from build123d import *

# Parameters (mm, degrees)
POCKET_DEPTH       = 5.2
POCKET001_DEPTH    = 131.2836295795
POLARPATTERN_COUNT = 3
SKETCH003_R        = 1.65
POCKET002_DEPTH    = 3.601


with BuildPart() as part:
    # Sketch → Revolution (revolve)
    with BuildSketch(Plane.XZ):
        Polygon((15.1, 0), (15.1, 3.9), (21.6, 3.9), (21.6, 1.7), (22.6, 1.7), (22.6, 0), align=None)
    revolve(axis=Axis((0, 0, 0), (0, 0, 1)))

    # Sketch001 → Pocket (cut)
    with BuildSketch(Plane.XY.offset(0.3)):
        with BuildLine():
            ThreePointArc((-15.9712383567, -3.8204989231), (-18.8447644437, -5.9331508585), (-16.9057454793, -8.9265863145))
            ThreePointArc((-16.1835232571, -10.1775118978), (-16.2776050381, -9.3978796505), (-16.9057454793, -8.9265863145))
            ThreePointArc((-16.1835232571, -10.1775118978), (-14.5606415898, -13.3534693073), (-11.2942683009, -11.9212486852))
            ThreePointArc((-9.7295516419, -11.5475462696), (-10.6061902717, -11.3396396422), (-11.2942683009, -11.9212486852))
            ThreePointArc((-9.7295516419, -11.5475462696), (0, -15.1), (9.7295516419, -11.5475462696))
            ThreePointArc((11.2942683009, -11.9212486852), (10.6061902717, -11.3396396422), (9.7295516419, -11.5475462696))
            ThreePointArc((11.2942683009, -11.9212486852), (14.5606415898, -13.3534693073), (16.1835232571, -10.1775118978))
            ThreePointArc((16.9057454793, -8.9265863145), (16.2776050381, -9.3978796505), (16.1835232571, -10.1775118978))
            ThreePointArc((16.9057454793, -8.9265863145), (18.8447644437, -5.9331508585), (15.9712383567, -3.8204989231))
            ThreePointArc((14.8652442418, -2.6522657545), (15.1235111358, -3.5154103916), (15.9712383567, -3.8204989231))
            ThreePointArc((14.8652442418, -2.6522657545), (13.0769835971, 7.55), (5.1356925999, 14.1998120241))
            ThreePointArc((4.6769700558, 15.7417476083), (4.517320864, 14.8550500338), (5.1356925999, 14.1998120241))
            ThreePointArc((4.6769700558, 15.7417476083), (4.2841228539, 19.2866201659), (0.7222222222, 19.1040982123))
            ThreePointArc((-0.7222222222, 19.1040982123), (0, 18.7957593011), (0.7222222222, 19.1040982123))
            ThreePointArc((-0.7222222222, 19.1040982123), (-4.2841228539, 19.2866201659), (-4.6769700558, 15.7417476083))
            ThreePointArc((-5.1356925999, 14.1998120241), (-4.517320864, 14.8550500338), (-4.6769700558, 15.7417476083))
            ThreePointArc((-5.1356925999, 14.1998120241), (-13.0769835972, 7.55), (-14.8652442418, -2.6522657545))
            ThreePointArc((-15.9712383567, -3.8204989231), (-15.1235111358, -3.5154103916), (-14.8652442418, -2.6522657545))
        make_face()
    extrude(amount=POCKET_DEPTH, mode=Mode.SUBTRACT)

    # Sketch002 → Pocket001 (cut, through all)
    with BuildSketch(Plane.XY.offset(0.7)):
        with BuildLine():
            Line((-21.1456411257, 3.728513813), (-19.8005265105, 3.4913338142))
            ThreePointArc((-19.8005265105, 3.4913338142), (-17.143892895, 3.9448230849), (-15.3779467169, 5.9806985187))
            ThreePointArc((-8.5602136605, 14.1057698155), (-12.6397419459, 10.6059852697), (-15.3779467169, 5.9806985187))
            ThreePointArc((-8.5602136605, 14.1057698155), (-6.8619255723, 16.1984130552), (-6.876646489, 18.8934309501))
            Line((-7.3438021199, 20.1769304973), (-6.876646489, 18.8934309501))
            ThreePointArc((-6.6329850074, 21.6047103635), (-7.2948567632, 21.0433924702), (-7.3438021199, 20.1769304973))
            ThreePointArc((-6.6329850074, 21.6047103635), (-17.3126154887, 14.5269867812), (-22.428296266, 2.7805622822))
            ThreePointArc((-21.1456411257, 3.728513813), (-21.9904400194, 3.5298512156), (-22.428296266, 2.7805622822))
        make_face()
    pocket001 = extrude(amount=POCKET001_DEPTH, mode=Mode.SUBTRACT)

    # PolarPattern: Pocket001 ×3 about axis
    polarpattern_axis = Axis((0, 0, 0.7), (0, 0, 1))
    for i in range(1, POLARPATTERN_COUNT):
        add(pocket001.rotate(polarpattern_axis, i * 360 / POLARPATTERN_COUNT), mode=Mode.SUBTRACT)

    # Sketch003 → Pocket002 (cut, through all)
    with BuildSketch(Plane.XY.offset(0.3)):
        with Locations((8.75, 15.1554445662)):
            Circle(SKETCH003_R)
        with Locations((-17.5, 0)):
            Circle(SKETCH003_R)
        with Locations((8.75, -15.1554445662)):
            Circle(SKETCH003_R)
    extrude(amount=POCKET002_DEPTH, mode=Mode.SUBTRACT)


solid = part.part
Can you work these out from the model? Positions are in its coordinate system, mm. A direction names the side the tool comes from. Give positions to 0.01 mm unless a question says otherwise; leave off trailing zeros. Loops run counter-clockwise (first coordinate to the right, second up) from the corner with the lowest first, then second, coordinate; pieces in that order, holes last. Notation, with made-up numbers: (64, -20.75) - (111, -20.75) arc R26 cw to (111, 2.25) - close; hole circle Ø11 at (70, 64). An arc over 180 degrees is marked (long way). Return JSON: item names as keys, results as strings.
1. I'm going to push flat-ended pins straight in: pin 1 Ø3 at (x, y) = (-17.5, 0) entering from +Z; pin 2 Ø3 at (x, y) = (18, 10.5) entering from +Z; pin 3 Ø2 at (y, z) = (-11, 2) entering from -X. Where does each tip first touch, or does it pass through?
Output values:
{"pin 1": "stops at z = 0.3", "pin 2": "stops at z = 0.7", "pin 3": "stops at x = -20.24"}
2. We'd pull the mould along X, two halves only. Please class faces 5 (the face through (10.619, -11.343, 2.075)), 6 (the face through (3.907, 21.244, 2.785)), 7 (the face through (-20.35, -7.24, 2.78)), 8 (the face through (15.115, -3.506, 2.075)): +X half, -X half, draft (parallel to the pull), parting line (faces both ways), or undercut.
Output values:
{"face 5": "undercut", "face 6": "parting line", "face 7": "-X half", "face 8": "undercut"}
3. I want a section at D-D on z = 2.3. Give the number of separate pieces and of enclosed holes in the cut face, and give its area (3 significant figures).
Output values:
{"separate pieces": "1", "enclosed holes": "4", "area": "297 mm²"}
4. For faces 1 (the face through (9, 15, 0.3)), 2 (the face through (14.056, 17.069, 1.211)), 3 (the face through (-20.48, 3.61, 2.28)), 4 (the face through (-7.363, 20.871, 1.211)), which set-ups out of +Z, -Z, +X, -X, +Y, -Y let a thin tool reach every point of the face, with its end or its side?
Output values:
{"face 1": "+Z", "face 2": "+Z, +X", "face 3": "+Z, +Y", "face 4": "+Z, -X"}
5. I want a section at A-A on x = 8. Please give me the cut outline in (y, z), and give its area (3 significant figures).
Output values:
{"outline": "(-21.14, 0) - (-12.81, 0) - (-12.81, 3.9) - (-13.69, 3.9) - (-13.69, 0.3) - (-16.63, 0.3) - (-16.63, 3.9) - (-20.06, 3.9) - (-20.06, 1.7) - (-20.83, 1.7) - (-20.83, 0.7) - (-21.14, 0.7) - close; (12.81, 0) - (21.14, 0) - (21.14, 1.7) - (20.06, 1.7) - (20.06, 3.9) - (16.63, 3.9) - (16.63, 0.3) - (13.69, 0.3) - (13.69, 3.9) - (12.81, 3.9) - close", "area": "38.8 mm²"}
6. I want a section at B-B on y = -6. Please give me the cut outline in (x, z), and give its area (3 significant figures).
Output values:
{"outline": "(-21.79, 0) - (-13.86, 0) - (-13.86, 0.3) - (-18.86, 0.3) - (-18.86, 3.9) - (-20.75, 3.9) - (-20.75, 1.7) - (-21.79, 1.7) - close; (13.86, 0) - (21.79, 0) - (21.79, 1.7) - (20.75, 1.7) - (20.75, 3.9) - (18.86, 3.9) - (18.86, 0.3) - (13.86, 0.3) - close", "area": "21.3 mm²"}
7. I want a section at C-C on x = -17.5. Please give me the cut outline in (y, z).
Output values:
{"outline": "(-14.3, 0) - (14.3, 0) - (14.3, 0.7) - (3.77, 0.7) - (3.77, 3.9) - (1.65, 3.9) - (1.65, 0.3) - (-1.65, 0.3) - (-1.65, 3.9) - (-4.1, 3.9) - (-4.1, 0.3) - (-8.7, 0.3) - (-8.7, 3.9) - (-12.66, 3.9) - (-12.66, 1.7) - (-14.3, 1.7) - close"}
8. If I drill on line 1 (X direction, y = 0, z = 2.1); line 2 (X direction, y = 16, z = 1.55); line 3 (Y direction, x = -17.5, z = 2.4), over which ranges is the centre line in solid material (lowest first)?
Output values:
{"line 1": "x = -21.6 to -19.15, -15.85 to -15.1, 15.1 to 16.52", "line 2": "x = -6.94 to -4.85, 4.85 to 7.33, 10.17 to 13.43", "line 3": "y = -12.66 to -8.7, -4.1 to -1.65, 1.65 to 3.77"}
